Source: CAD feature listing. Evaluate the final solid. Frame: model axes, mm. Coordinates: 2 decimals unless noted, no trailing zeros. Order: outer loops, then holes, each group sorted by start corner. A loop starts at its lowest first (then second) coordinate and runs counter-clockwise, first axis right, second up. Notation, with made-up numbers: (-36, 56) -> (14, 56) arc R16 cw to (14, 85) -> close; hole circle Ø11 at (30.5, 23). An arc over 180 degrees is marked (long way). Write each question's results on one line, items separated by ' | '. Start each with the question number.
from build123d import *

# Parameters (mm, degrees)
F0_R     = 4
F1_DEPTH = 2.5
F3_DEPTH = 5


# Not quite as in the source:
# - a feature names something its author has since deleted; it is built from what else it names


with BuildPart() as f1:
    # F0 (on Front) → F1 (new body, symmetric)
    with BuildSketch(Plane.XZ):
        with BuildLine():
            Line((-58.4079127312, -18.8516896643), (-58.4079127312, -113.2025790236))
            ThreePointArc((-58.4079127312, -113.2025790236), (-60.3576601995, -124.4768818123), (-49.0833574108, -122.527134344))
            Line((-49.0833574108, -122.527134344), (43.2675319485, -122.527134344))
            ThreePointArc((43.2675319485, -122.527134344), (54.5418347371, -124.4768818123), (52.5920872688, -113.2025790236))
            Line((52.5920872688, -113.2025790236), (52.5920872688, -18.8516896643))
            ThreePointArc((52.5920872688, -18.8516896643), (56.5920872688, -12.527134344), (52.5920872688, -6.2025790236))
            Line((52.5920872688, -6.2025790236), (52.5920872688, 21.8966218341))
            ThreePointArc((52.5920872688, 21.8966218341), (58.408131243, 32.1608112925), (52.5920872688, 42.425000751))
            Line((52.5920872688, 42.425000751), (52.5920872688, 88.1483103357))
            ThreePointArc((52.5920872688, 88.1483103357), (54.5418347371, 99.4226131243), (43.2675319485, 97.472865656))
            Line((43.2675319485, 97.472865656), (-49.0833574108, 97.472865656))
            ThreePointArc((-49.0833574108, 97.472865656), (-60.3576601995, 99.4226131243), (-58.4079127312, 88.1483103357))
            Line((-58.4079127312, 88.1483103357), (-58.4079127312, -6.2025790236))
            ThreePointArc((-58.4079127312, -6.2025790236), (-62.4079127312, -12.527134344), (-58.4079127312, -18.8516896643))
        make_face()
        with Locations((-55.4079127312, -119.527134344)):
            Circle(F0_R, mode=Mode.SUBTRACT)
        with Locations((49.5920872688, -119.527134344)):
            Circle(F0_R, mode=Mode.SUBTRACT)
        with Locations((-55.4079127312, -12.527134344)):
            Circle(F0_R, mode=Mode.SUBTRACT)
        with Locations((-55.4079127312, 94.472865656)):
            Circle(F0_R, mode=Mode.SUBTRACT)
        with Locations((49.5920872688, -12.527134344)):
            Circle(F0_R, mode=Mode.SUBTRACT)
        with Locations((49.5920872688, 94.472865656)):
            Circle(F0_R, mode=Mode.SUBTRACT)
    extrude(amount=F1_DEPTH, both=True)

    # F2 (on Front) → F3 (cut, symmetric)
    with BuildSketch(Plane.XZ):
        with BuildLine():
            Line((40.5920872688, 85.472865656), (-46.4079127312, 85.472865656))
            Line((-46.4079127312, 85.472865656), (-46.4079127312, -110.527134344))
            Line((-46.4079127312, -110.527134344), (40.5920872688, -110.527134344))
            Line((40.5920872688, -110.527134344), (40.5920872688, 21.8337872246))
            ThreePointArc((40.5920872688, 21.8337872246), (47.5920872688, 32.7424993392), (40.5920872688, 43.6512114539))
            Line((40.5920872688, 43.6512114539), (40.5920872688, 85.472865656))
        make_face()
    extrude(amount=F3_DEPTH, both=True, mode=Mode.SUBTRACT)


solid = f1.part
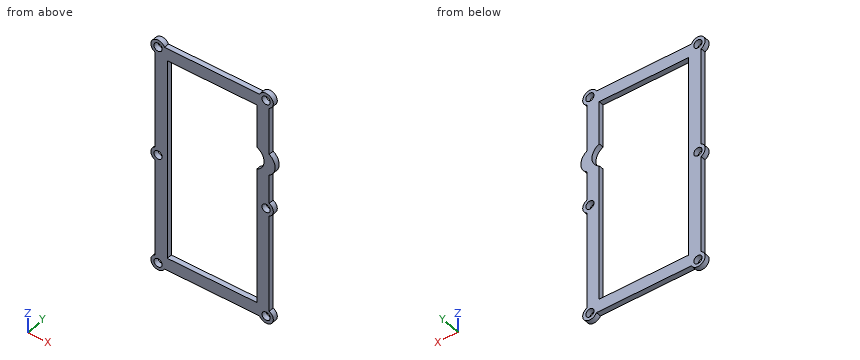
(1) Section C-C on y = -0.9. Return the cut outline in (x, z) (1 decimal), then the cut area to 3 significant figures.
(2) First-contact query: P1, Ø1.5, axis at x = -8, y = 1, coming from the -Z side; P2, Ø2.5, axis at x = -21.5, y = 0.5, coming from the +Z side; P3, Ø6.5, axis at x = 49.59, z = -119.53, coming from the +Y side; P4, Ø5, axis at x = 40, z = 54.5, coming from the +Y side. Flat tips, straight axial feed; report the tip coordinate or a pass-through.
(3) Line query: L1, parallel to Z at x = 8.5, y = 1.1; L2, parallel to Z at x = -56, y = 0.95; L3, parallel to X at y = 2, z = -72. Output: solid intervals per line, ascending.
(4) Section D-D on x = -54. Return the cut outline in (y, z).
(5) Section A-A on z = 51. Return the cut outline in (x, y), then the cut area to 3 significant figures.
(6) Section B-B on x = 16.5. Return the cut outline in (y, z).
Results list:
1) outline: (-58.4, -113.2) arc R7 ccw (long way) to (-49.1, -122.5) -> (43.3, -122.5) arc R7 ccw (long way) to (52.6, -113.2) -> (52.6, -18.9) arc R7 ccw to (52.6, -6.2) -> (52.6, 21.9) arc R12 ccw to (52.6, 42.4) -> (52.6, 88.1) arc R7 ccw (long way) to (43.3, 97.5) -> (-49.1, 97.5) arc R7 ccw (long way) to (-58.4, 88.1) -> (-58.4, -6.2) arc R7 ccw to (-58.4, -18.9) -> close; hole circle Ø8 at (-55.4, -119.5); hole circle Ø8 at (-55.4, -12.5); hole circle Ø8 at (-55.4, 94.5); hole (-46.4, -110.5) -> (40.6, -110.5) -> (40.6, 21.8) arc R12 ccw to (40.6, 43.7) -> (40.6, 85.5) -> (-46.4, 85.5) -> close; hole circle Ø8 at (49.6, -119.5); hole circle Ø8 at (49.6, -12.5); hole circle Ø8 at (49.6, 94.5) | area: 7,380 mm²
2) P1: stops at z = -122.53 | P2: stops at z = 97.47 | P3: passes through | P4: stops at y = 2.5
3) L1: z = -122.53 to -110.53, 85.47 to 97.47 | L2: z = -126.5 to -123.48, -115.57 to -16.48, -8.57 to 90.52, 98.43 to 101.45 | L3: x = -58.41 to -46.41, 40.59 to 52.59
4) outline: (-2.5, -126.38) -> (2.5, -126.38) -> (2.5, -123.27) -> (-2.5, -123.27) -> close; (-2.5, -115.78) -> (2.5, -115.78) -> (2.5, -16.27) -> (-2.5, -16.27) -> close; (-2.5, -8.78) -> (2.5, -8.78) -> (2.5, 90.73) -> (-2.5, 90.73) -> close; (-2.5, 98.22) -> (2.5, 98.22) -> (2.5, 101.33) -> (-2.5, 101.33) -> close
5) outline: (-58.41, -2.5) -> (-46.41, -2.5) -> (-46.41, 2.5) -> (-58.41, 2.5) -> close; (40.59, -2.5) -> (52.59, -2.5) -> (52.59, 2.5) -> (40.59, 2.5) -> close | area: 120 mm²
6) outline: (-2.5, -122.53) -> (2.5, -122.53) -> (2.5, -110.53) -> (-2.5, -110.53) -> close; (-2.5, 85.47) -> (2.5, 85.47) -> (2.5, 97.47) -> (-2.5, 97.47) -> close
